The model under review builds one solid part; all positions refer to its coordinate system, in mm. A direction names the side the tool comes from. Give positions to 0.01 mm unless a question says otherwise; leave off trailing zeros. Order: outer loops, then holes, each group sorted by start corner. A loop starts at its lowest first (then second) coordinate and runs counter-clockwise, first axis right, second up. Notation, with made-up numbers: (57, 84) - (72, 84) arc R27 ccw to (72, 123) - close; hole circle Ø2 at (88.5, 68.5). An arc over 180 degrees is marked (long way). Use CSV: the item, a comma, the result in double quotes.
Autodesk Inventor part; units mm, degrees
ref_plane "YZ Plane" through (0, 0, 0) normal (1, 0, 0) x (0, 1, 0)
ref_plane "XZ Plane" through (0, 0, 0) normal (0, 1, 0) x (-1, 0, 0)
ref_plane "XY Plane" through (0, 0, 0) normal (0, 0, 1) x (1, 0, 0)
sketch "Esquisse3" plane through (0, 0, 0) normal (0, 1, 0) x (-1, 0, 0)
  line L0 (-0.25, 6.0789) -> (-0.25, -5.5)
  line L1 (-8, 10) -> (-8, -4)
  line L2 (-8, -4) -> (-5.5, -4)
  line L3 (-5.5, -4) -> (-3, 10)
  line L4 (-3, 10) -> (-8, 10)
  line L5 (0, -31.6) -> (0, 151.1) construction
  line L6 (5.05, 0) -> (-30.3, 0) construction
  line L7 (-3, 10) -> (-20.25, 25)
  line L8 (-20.25, 25) -> (-20.25, 125)
  line L9 (-8, 10) -> (-25.25, 25)
  line L10 (-25.25, 25) -> (-25.25, 125)
  line L11 (-25.25, 125) -> (-20.25, 125)
  line L12 (-30.3, 0) -> (5.05, 0) construction
  point P0 (0, 0)
  dimension "d0" = 5.5
  dimension "d1" = 10.5
  dimension "d2" = 15.5
  dimension "d3" = 14
  dimension "d4" = 8
  dimension "d5" = 10
  dimension "d9" = 40
  dimension "d10" = 15
  dimension "d11" = 100
  dimension "d13" = 5
  dimension "d14" = 5
  dimension "d15" = 125
revolve "Révolution1" add sketch "Esquisse3" angle 360 about axis through (0.25, 0, 6.0789) along (0, 0, -1)
properties part number "P006_CanonConfettis"
Item 1: Mouldability with a two-part tool opening along Y and no side actions: class faces 1 (the face through (8.671, 2.652, 10.938)), 2 (the face through (-2, 5, -4)), 3 (the face through (19.326, 6.007, 75.7)) as pulls with the +Y half, pulls with the -Y half, needs draft (parallel to the pull), parting line crosses it, or undercut.
Results list:
face 1,"parting line crosses it"
face 2,"needs draft"
face 3,"undercut"
Item 2: Wall thickness on L1, parallel to Y at x = 0.25, z = 78.5; L2, parallel to X at y = 0, z = 73; L3, parallel to Y at x = -11, z = 91.5: over which ranges is each line inside the solid? List them lowest first.
Results list:
L1,"y = -25 to -20, 20 to 25"
L2,"x = -24.75 to -19.75, 20.25 to 25.25"
L3,"y = -22.33 to -16.54, 16.54 to 22.33"
Item 3: Take a section at B-B, the plane y = 0. Give the boundary of the cut face in (x, z), and give its area (4 significant figures).
Results list:
outline,"(-24.75, 25) - (-7.5, 10) - (-7.5, -4) - (-5, -4) - (-2.5, 10) - (-19.75, 25) - (-19.75, 125) - (-24.75, 125) - close; (3, 10) - (5.5, -4) - (8, -4) - (8, 10) - (25.25, 25) - (25.25, 125) - (20.25, 125) - (20.25, 25) - close"
area,"1,255 mm2"
Item 4: Take a section at A-A, the plane x = 0.25. Give the boundary of the cut face in (y, z), and give its area (4 significant figures).
Results list:
outline,"(-25, 25) - (-7.75, 10) - (-7.75, -4) - (-5.25, -4) - (-2.75, 10) - (-20, 25) - (-20, 125) - (-25, 125) - close; (2.75, 10) - (5.25, -4) - (7.75, -4) - (7.75, 10) - (25, 25) - (25, 125) - (20, 125) - (20, 25) - close"
area,"1,255 mm2"
Item 5: Take a section at C-C, the plane z = 68. Give the boundary of the cut face in (x, y).
Results list:
outline,"circle Ø50 at (0.25, 0); hole circle Ø40 at (0.25, 0)"
Item 6: Tool access review of faces 4 (the face through (-0.759, -7.684, 2.902)), 5 (the face through (-4.3, -3.5, 12.6)): name each direction out of +Z, -Z, +X, -X, +Y, -Y from which nothing blocks a thin tool from reaching the whole face with its end or side.
Results list:
face 4,"-Z"
face 5,"+Z"
Item 7: Clearance check with flat-ended pins moving along their axes: pin 1 (1.5 mm diameter, centred on x = -12.5, z = 23.5, fed in from -Y); pin 2 (5 mm diameter, centred on y = -13, z = 49.5, fed in from +X); pin 3 (1.5 mm diameter, centred on y = 5, z = 80, fed in from -X). State where each tip first meets the part, or that it passes through.
Results list:
pin 1,"stops at y = -20.59"
pin 2,"stops at x = 22.94"
pin 3,"stops at x = -24.39"
